from build123d import *

# Parameters (mm, degrees)
F0_W     = 527.05
F0_H     = 400.05
F0_W_2   = 514.35
F0_H_2   = 387.35
F1_DEPTH = 177.8
F2_W     = 527.05
F2_H     = 400.05
F3_DEPTH = 6.35
F4_R     = 12.7


with BuildPart() as f1:
    # F0 (on Top) → F1 (new body)
    with BuildSketch(Plane.XY):
        Rectangle(F0_W, F0_H)
        Rectangle(F0_W_2, F0_H_2, mode=Mode.SUBTRACT)
    extrude(amount=F1_DEPTH)

    # F2 (on face) → F3 (join)
    with BuildSketch(Plane(origin=(0, 0, 0), x_dir=(1, 0, 0), z_dir=(0, 0, -1))):
        Rectangle(F2_W, F2_H)
    extrude(amount=F3_DEPTH)

    # F4
    f4_edges = [f1.edges().sort_by_distance(p)[0] for p in [
        (0, 193.675, 0),
        (-257.175, 0, 0),
        (0, -193.675, 0),
        (257.175, 0, 0),
        (-257.175, 193.675, 88.9),
        (-257.175, -193.675, 88.9),
        (257.175, -193.675, 88.9),
        (257.175, 193.675, 88.9),
    ]]
    fillet(f4_edges, radius=F4_R)


solid = f1.part
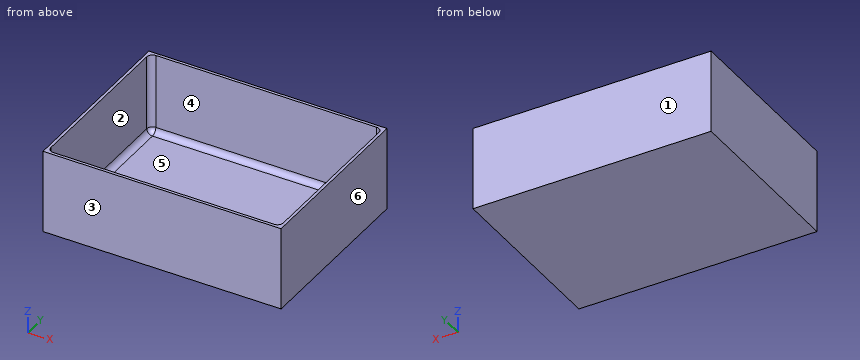
CAD build for the part. Positions are in the model's coordinates, mm. Face numbers are marked on the shaded views. A direction names the side the tool comes from. Coordinates: 2 decimals unless noted, no trailing zeros. Write each loop counter-clockwise with the first axis right and the second up, starting at its lowest first coordinate (ties: lowest second). Pieces come first, ordered by that corner, then holes. Notation, with made-up numbers: (36.25, 17) - (42.25, 17) arc R7 ccw to (42.25, 23) - close; hole circle Ø7 at (8, 45.25). An arc over 180 degrees is marked (long way). Use a Markdown table: item, result. Add a question column.
Item 1: Mould opens along X. For the marked faces 3, 4, 5 and 6 say: pulls with the +X half, pulls with the -X half, needs draft (parallel to the pull), parting line crosses it, or undercut.
Item 2: Flat gauge pin, fed straight in: pin 1 (10 mm diameter, centred on x = 104, y = -66.5, fed in from +Z). Where does the tip first touch, or does it go through?
Item 3: Drill centre lines: L1, parallel to X at y = 4, z = 78 (3 decimals); L2, parallel to Y at x = 228.5, z = 165 (3 decimals); L3, parallel to Z at x = 202, y = 151. Where is each one in solid material? Low to high. Write a range as from..to.
Item 4: 3-axis set-ups, long thin cutter, end or side, ignore diameter. For the marked faces 1 and 2: which of +Z, -Z, +X, -X, +Y, -Y reach the whole face in a straight line?
Item 5: Band-saw the part on A-A, the plane z = 29. Give the cut face in (x, y) (3 decimals).
Item 6: Band-saw the part on B-B, the plane y = -7.5. Give the cut face in (x, z) (3 decimals).
Item 7: Band-saw the part on C-C, the plane x = 206.5. Give the cut face in (y, z) (3 decimals), and give its area (3 significant figures).
Numbers:
| question | item | result |
|---|---|---|
| 1 | face 3 | needs draft |
| 1 | face 4 | undercut |
| 1 | face 5 | undercut |
| 1 | face 6 | pulls with the +X half |
| 2 | pin 1 | z = 0 |
| 3 | L1 | -263.525..-257.175, 257.175..263.525 |
| 3 | L2 | -200.025..-193.675, 193.675..200.025 |
| 3 | L3 | -6.35..0 |
| 4 | face 1 | +Z, -Z, +X, -X, +Y |
| 4 | face 2 | +Z |
| 5 | outline | (-263.525, -200.025) - (263.525, -200.025) - (263.525, 200.025) - (-263.525, 200.025) - close; hole (-257.175, -180.975) arc R12.7 ccw to (-244.475, -193.675) - (244.475, -193.675) arc R12.7 ccw to (257.175, -180.975) - (257.175, 180.975) arc R12.7 ccw to (244.475, 193.675) - (-244.475, 193.675) arc R12.7 ccw to (-257.175, 180.975) - close |
| 6 | outline | (-263.525, -6.35) - (263.525, -6.35) - (263.525, 177.8) - (257.175, 177.8) - (257.175, 12.7) arc R12.7 cw to (244.475, 0) - (-244.475, 0) arc R12.7 cw to (-257.175, 12.7) - (-257.175, 177.8) - (-263.525, 177.8) - close |
| 7 | outline | (-200.025, -6.35) - (200.025, -6.35) - (200.025, 177.8) - (193.675, 177.8) - (193.675, 12.7) arc R12.7 cw to (180.975, 0) - (-180.975, 0) arc R12.7 cw to (-193.675, 12.7) - (-193.675, 177.8) - (-200.025, 177.8) - close |
| 7 | area | 4,870 mm2 |
